The model under review builds one solid part; all positions refer to its coordinate system, in mm. Give positions to 0.01 mm unless a question says otherwise; leave off trailing zeros. Order: outer loops, then holes, each group sorted by start corner. A loop starts at its lowest first (then second) coordinate and runs counter-clockwise, first axis right, second up. Notation, with made-up numbers: (42.5, 61) - (87.5, 61) arc R22 ccw to (87.5, 67) - close; hole circle Ø9 at (67.5, 2). An arc over 180 degrees is marked (long way). Put each result on its own line as item: value.
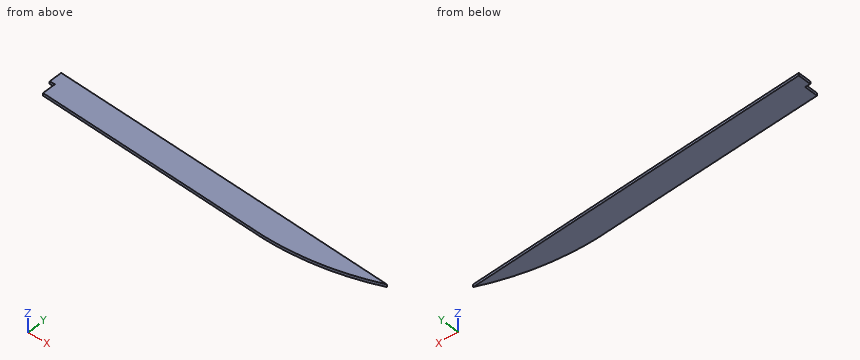
```python
from build123d import *

# Parameters (mm, degrees)
BOSS_EXTRUDE1_DEPTH = 10


with BuildPart() as part:
    # Sketch1 → Boss-Extrude1 (new body)
    with BuildSketch(Plane.XY):
        with BuildLine():
            Line((8e-09, 1e-09), (8e-09, -50.121840767))
            Line((8e-09, -50.121840767), (20.000000008, -50.121840767))
            Line((20.000000008, -50.121840767), (20.000000008, -101.641774289))
            ThreePointArc((20.000000008, -101.641774289), (465.566882769, -133.179218179), (911.080534453, -165.459917439))
            add(Edge.make_bspline(
                [(1319.077974178, -95.398302795), (1125.124112684, -174.190190217), (911.080534453, -165.459917439)],
                knots=[0, 0, 0, 1, 1, 1], degree=2))
            ThreePointArc((1319.077974178, -95.398302795), (659.597864045, -46.885056293), (8e-09, 1e-09))
        make_face()
    extrude(amount=BOSS_EXTRUDE1_DEPTH)


solid = part.part
```
(1) Clearance check with flat-ended pins moving along their axes: pin 1 Ø4 at (x, z) = (413.5, 5.5) entering from +Y; pin 2 Ø1 at (y, z) = (-90, 6) entering from -X. State where each tip first meets the part, or that it passes through.
The answers:
pin 1: y = -29.06
pin 2: x = 20
(2) Take a section at B-B, the plane x = 583.5. Write out the cut boundary in (y, z), then the cut area to 3 significant figures.
The answers:
outline: (-141.65, 0) - (-41.39, 0) - (-41.39, 10) - (-141.65, 10) - close
area: 1,000 mm^2
(3) Wall thickness on L1, parallel to Y at x = 515, z = 3.5; L2, parallel to Y at x = 1153, z = 3.5: over which ranges is each line inside the solid? List them lowest first.
The answers:
L1: -136.72 to -36.47
L2: -146.06 to -83.03
